Part model, mm, in its own coordinate system. Give positions to 0.01 mm unless a question says otherwise; leave off trailing zeros. Write each loop counter-clockwise with the first axis right and the second up, starting at its lowest first coordinate (ties: lowest second). Pieces come first, ordered by that corner, then holes. Notation, with made-up numbers: M 30,30 L 44,30 A8 cw 44,40 Z; hole C 15.25,-8.75 d6. An arc over 180 degrees is marked long. Use a Markdown table: item, result.
Autodesk Inventor part; units mm, degrees
ref_plane "Work Plane32" through (254, 330.2, 0) normal (0, 0, -1) x (-1, 0, 0)
ref_plane "Work Plane28" through (254, 330.2, -6.35) normal (0, 0, -1) x (-1, 0, 0)
ref_plane "YZ Plane" through (0, 0, 0) normal (1, 0, 0) x (0, 1, 0)
ref_plane "Work Plane32" through (254, 330.2, 0) normal (0, 0, -1) x (-1, 0, 0)
sketch "Sketch36" plane through (254, 330.2, 0) normal (0, 0, -1) x (-1, 0, 0)
  line L0 (254, -363.855) -> (254, -196.85)
  line L1 (0, 0) -> (0, -114.3)
  line L2 (254, -363.855) -> (0, -363.855)
  line L3 (0, -363.855) -> (0, 0)
  line L4 (0, 0) -> (254, 0)
  line L5 (254, 0) -> (254, -363.855)
  line L6 (342.9, -196.85) -> (342.9, -114.3)
  line L7 (342.9, -196.85) -> (254, -196.85)
  line L8 (254, -196.85) -> (254, -114.3)
  line L9 (254, -114.3) -> (342.9, -114.3)
  line L10 (342.9, -114.3) -> (342.9, -196.85)
  line L11 (-31.75, -363.855) -> (254, -363.855)
  line L12 (0, -314.325) -> (0, -196.85)
  line L13 (-31.75, -363.855) -> (0, -363.855)
  line L14 (0, -363.855) -> (0, -314.325)
  line L15 (0, -314.325) -> (-31.75, -314.325)
  line L16 (-31.75, -314.325) -> (-31.75, -363.855)
  line L17 (0, -196.85) -> (-88.9, -196.85)
  line L18 (-88.9, -196.85) -> (-88.9, -114.3)
  line L19 (-88.9, -114.3) -> (0, -114.3)
  line L20 (0, -114.3) -> (0, -196.85)
  dimension "d412" = 82.55
  dimension "d413" = 254
  dimension "d414" = 31.75
extrude "Extrusion20" add sketch "Sketch36" along normal blind 6.35
ref_plane "Work Plane28" through (254, 330.2, -6.35) normal (0, 0, -1) x (-1, 0, 0)
sketch "Sketch38" plane through (254, 330.2, -6.35) normal (0, 0, -1) x (-1, 0, 0)
  circle A0 centre (273.685, -183.515) radius 1.778
  circle A1 centre (273.685, -183.515) radius 1.778
  circle A2 centre (339.725, -183.515) radius 1.778
  circle A3 centre (339.725, -183.515) radius 1.778
  circle A4 centre (339.725, -117.475) radius 1.778
  circle A5 centre (339.725, -117.475) radius 1.778
  circle A6 centre (273.685, -117.475) radius 1.778
  circle A7 centre (273.685, -117.475) radius 1.778
  circle A8 centre (263.1059, -119.0625) radius 1.778
  circle A9 centre (263.1059, -119.0625) radius 1.778
  circle A10 centre (107.95, -332.105) radius 1.905
  circle A11 centre (107.95, -332.105) radius 1.905
  circle A12 centre (107.95, -322.58) radius 1.905
  circle A13 centre (107.95, -322.58) radius 1.905
  circle A14 centre (107.95, -303.53) radius 1.905
  circle A15 centre (107.95, -303.53) radius 1.905
  circle A16 centre (107.95, -357.505) radius 1.905
  circle A17 centre (107.95, -357.505) radius 1.905
  circle A18 centre (146.05, -303.53) radius 1.905
  circle A19 centre (146.05, -303.53) radius 1.905
  circle A20 centre (146.05, -322.58) radius 1.905
  circle A21 centre (146.05, -322.58) radius 1.905
extrude "Extrusion21" cut sketch "Sketch38" against normal blind 6.35
sketch "Sketch39" plane through (254, 330.2, -6.35) normal (0, 0, -1) x (-1, 0, 0)
  line L0 (0, -196.85) -> (0, -314.325)
  line L1 (0, -196.85) -> (5.08, -196.85)
  line L2 (5.08, -196.85) -> (5.08, -314.325)
  line L3 (5.08, -314.325) -> (0, -314.325)
  line L4 (0, -314.325) -> (0, -196.85)
  line L5 (254, -363.855) -> (254, -196.85)
  line L6 (-31.75, -363.855) -> (254, -363.855)
  line L7 (254, -196.85) -> (248.92, -196.85)
  line L8 (248.92, -196.85) -> (248.92, -363.855)
  line L9 (248.92, -363.855) -> (254, -363.855)
  line L10 (254, -363.855) -> (254, -196.85)
  line L11 (0, -114.3) -> (-88.9, -114.3)
  line L12 (254, 0) -> (0, 0)
  line L13 (0, -114.3) -> (5.08, -114.3)
  line L14 (5.08, -114.3) -> (5.08, 0)
  line L15 (5.08, 0) -> (0, 0)
  line L16 (0, 0) -> (0, -114.3)
  line L17 (254, 0) -> (248.92, 0)
  line L18 (248.92, 0) -> (248.92, -114.3)
  line L19 (248.92, -114.3) -> (254, -114.3)
  line L20 (254, -114.3) -> (254, 0)
  point P0 (254, -330.2)
  dimension "d415" = 5.08
  dimension "d416" = 5.08
  dimension "d417" = 5.08
extrude "Extrusion22" cut sketch "Sketch39" against normal blind 6.35
sketch "Sketch40" plane through (254, 330.2, -6.35) normal (0, 0, -1) x (-1, 0, 0)
  line L0 (5.08, 0) -> (5.08, -114.3)
  line L1 (248.92, 0) -> (5.08, 0)
  line L2 (248.92, -114.3) -> (248.92, 0)
  line L3 (-31.75, -363.855) -> (248.92, -363.855)
  line L4 (248.92, -363.855) -> (248.92, -196.85)
  circle A0 centre (11.43, -305.435) radius 1.778
  circle A1 centre (11.43, -267.335) radius 1.778
  circle A2 centre (11.43, -229.235) radius 1.778
  circle A3 centre (11.43, -82.55) radius 1.778
  circle A4 centre (11.43, -44.45) radius 1.778
  circle A5 centre (11.43, -6.35) radius 1.778
  circle A6 centre (242.57, -6.35) radius 1.778
  circle A7 centre (242.57, -44.45) radius 1.778
  circle A8 centre (242.57, -82.55) radius 1.778
  circle A9 centre (242.57, -229.235) radius 1.778
  circle A10 centre (242.57, -267.335) radius 1.778
  circle A11 centre (242.57, -305.435) radius 1.778
  point P0 (254, -330.2)
  dimension "d420" = 6.35
  dimension "d421" = 6.35
  dimension "d422" = 38.1
  dimension "d423" = 38.1
  dimension "d424" = 6.35
  dimension "d425" = 6.35
  dimension "d426" = 38.1
  dimension "d427" = 38.1
  dimension "d428" = 58.42
  dimension "d429" = 38.1
  dimension "d430" = 38.1
  dimension "d431" = 6.35
  dimension "d432" = 6.35
  dimension "d433" = 6.35
  dimension "d434" = 3.556
  dimension "d435" = 3.556
  dimension "d436" = 3.556
  dimension "d437" = 3.556
  dimension "d438" = 3.556
  dimension "d439" = 3.556
  dimension "d440" = 3.556
  dimension "d441" = 3.556
  dimension "d442" = 3.556
  dimension "d443" = 3.556
  dimension "d444" = 3.556
  dimension "d445" = 3.556
extrude "Extrusion23" cut sketch "Sketch40" against normal blind 6.35
sketch "Sketch41" plane through (254, 330.2, 0) normal (0, 0, 1) x (1, 0, 0)
  line L0 (-5.08, -314.325) -> (31.75, -314.325)
  line L1 (31.75, -363.855) -> (-248.92, -363.855)
  line L2 (31.75, -314.325) -> (-5.08, -314.325)
  line L3 (-5.08, -314.325) -> (-5.08, -363.855)
  line L4 (-5.08, -363.855) -> (31.75, -363.855)
  line L5 (31.75, -363.855) -> (31.75, -314.325)
  point P0 (-254, -330.2)
  dimension "d448" = 36.83
extrude "Extrusion24" cut sketch "Sketch41" against normal blind 6.35
properties part number "mark-2 plate"
1. Cut at B-B, the plane x = -27. Give the cut face in (y, z), then the cut area to 3 significant figures.
Findings below:
| item | result |
|---|---|
| outline | M 133.35,-6.35 L 215.9,-6.35 L 215.9,0 L 133.35,0 Z |
| area | 524 mm2 |
2. Cut at C-C, the plane z = -4. State how many separate pieces and enclosed holes the cut face has, then the cut area to 3 significant figures.
Findings below:
| item | result |
|---|---|
| separate pieces | 1 |
| enclosed holes | 23 |
| area | 104,000 mm2 |
3. Cut at A-A, the plane y = 222. Give the cut face in (x, z).
Findings below:
| item | result |
|---|---|
| outline | M 5.08,-6.35 L 248.92,-6.35 L 248.92,0 L 5.08,0 Z |
4. Drop flat-ended pins along their axis: P1, Ø3, axis at y = 39.5, z = -3, coming from the +X side; P2, Ø1.9, axis at x = -56.5, z = -2, coming from the -Y side; P3, Ø3, axis at y = 21.5, z = -5, coming from the -X side. Give the stop position or say it passes through.
Findings below:
| item | result |
|---|---|
| P1 | x = 248.92 |
| P2 | y = 133.35 |
| P3 | x = 5.08 |
5. Drill centre lines: L1, parallel to Y at x = 146.05, z = -3.75 (3 decimals); L2, parallel to X at y = 7, z = -4.75; L3, parallel to Y at x = -36, z = -2.5. Where is each one in solid material? Low to high.
Findings below:
| item | result |
|---|---|
| L1 | -33.655 to -29.21, -25.4 to -3.81, 0 to 5.715, 9.525 to 24.765, 28.575 to 330.2 |
| L2 | 5.08 to 106.15, 109.75 to 144.25, 147.85 to 248.92 |
| L3 | 133.35 to 215.9 |
